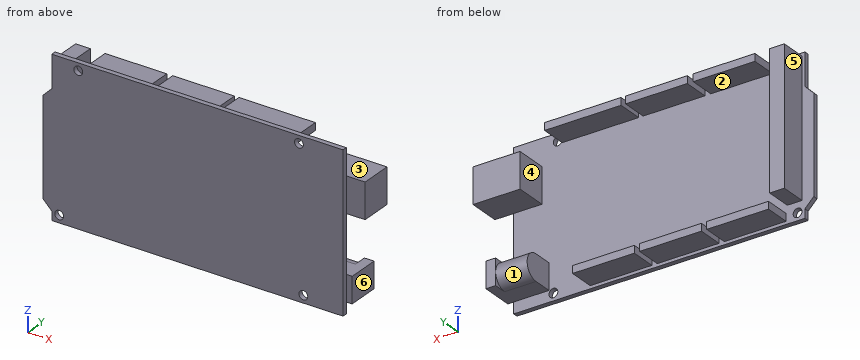
Autodesk Inventor part; units mm, degrees
ref_plane "YZ Plane" through (0, 0, 0) normal (1, 0, 0) x (0, 1, 0)
ref_plane "XZ Plane" through (0, 0, 0) normal (0, 1, 0) x (-1, 0, 0)
ref_plane "XY Plane" through (0, 0, 0) normal (0, 0, 1) x (1, 0, 0)
sketch "Sketch1" plane through (0, 0, 0) normal (0, 1, 0) x (-1, 0, 0)
  line L0 (0, 0) -> (99, 0)
  line L1 (99, 0) -> (99, 3)
  line L2 (99, 3) -> (102, 6)
  line L3 (102, 6) -> (102, 39)
  line L4 (102, 39) -> (99, 42)
  line L5 (99, 42) -> (99, 53)
  line L6 (99, 53) -> (0, 53)
  line L7 (0, 53) -> (0, 0)
  dimension "d0" = 99
  dimension "d1" = 3
  dimension "d2" = 135
  dimension "d3" = 33
  dimension "d4" = 3
  dimension "d5" = 3
  dimension "d6" = 53
extrude "Extrusion1" add sketch "Sketch1" along normal blind 1.6
sketch "Sketch2" plane through (0, 1.6, 0) normal (0, 1, 0) x (1, 0, 0)
  line L0 (0, 0) -> (-99, 0)
  line L1 (0, -53) -> (0, 0)
  line L2 (2, -3.8) -> (-12, -3.8)
  line L3 (-12, -3.8) -> (-12, -12.6)
  line L4 (-12, -12.6) -> (2, -12.6)
  line L5 (2, -12.6) -> (2, -3.8)
  dimension "d9" = 8.8
  dimension "d10" = 2
  dimension "d11" = 3.8
  dimension "d12" = 14
extrude "Extrusion2" add sketch "Sketch2" along normal blind 10.8
sketch "Sketch3" plane through (-12, 1.6, 3.8) normal (-1, 0, 0) x (0, 0, 1)
  line L0 (8.8, 0) -> (0, 0)
  line L1 (8.8, 0) -> (8.8, 10.8)
  line L2 (0, 10.8) -> (8.8, 10.8)
  line L3 (0, 0) -> (0, 10.8)
  arc A0 (8.8, 6.4) -> (0, 6.4) centre (4.4, 6.4) ccw
  point P0 (-3.8, -1.6)
extrude "Extrusion3" cut sketch "Sketch3" against normal blind 10.7 contours A0 L2 L1 | L3 L2 A0
sketch "Sketch4" plane through (0, 1.6, 0) normal (0, 1, 0) x (1, 0, 0)
  line L0 (-99, -53) -> (0, -53)
  line L1 (0, -53) -> (0, -12.6)
  line L2 (-9.6, -32) -> (6.4, -32)
  line L3 (6.4, -32) -> (6.4, -44)
  line L4 (6.4, -44) -> (-9.6, -44)
  line L5 (-9.6, -44) -> (-9.6, -32)
  dimension "d17" = 16
  dimension "d18" = 12
  dimension "d19" = 6.4
  dimension "d20" = 9
extrude "Extrusion4" add sketch "Sketch4" along normal blind 10.8
sketch "Sketch5" plane through (0, 1.6, 0) normal (0, 1, 0) x (1, 0, 0)
  line L0 (0, -3.8) -> (0, 0)
  line L1 (0, 0) -> (-99, 0)
  line L2 (-26, -3.5) -> (-47, -3.5)
  line L3 (-47, -3.5) -> (-47, -1)
  line L4 (-47, -1) -> (-26, -1)
  line L5 (-26, -1) -> (-26, -3.5)
  line L6 (-48.8, -3.5) -> (-69.8, -3.5)
  line L7 (-69.8, -3.5) -> (-69.8, -1)
  line L8 (-69.8, -1) -> (-48.8, -1)
  line L9 (-48.8, -1) -> (-48.8, -3.5)
  line L10 (-71.6, -3.5) -> (-92.6, -3.5)
  line L11 (-92.6, -3.5) -> (-92.6, -1)
  line L12 (-92.6, -1) -> (-71.6, -1)
  line L13 (-71.6, -1) -> (-71.6, -3.5)
  dimension "d23" = 21
  dimension "d24" = 2.5
  dimension "d25" = 26
  dimension "d26" = 1
  dimension "d29" = 22.8
extrude "Extrusion5" add sketch "Sketch5" along normal blind 8.7
sketch "Sketch6" plane through (0, 1.6, 0) normal (0, 1, 0) x (1, 0, 0)
  line L0 (0, 0) -> (-99, 0)
  line L1 (-102, -6) -> (-102, -39)
  line L2 (-98, -6) -> (-93, -6)
  line L3 (-93, -6) -> (-93, -52)
  line L4 (-93, -52) -> (-98, -52)
  line L5 (-98, -52) -> (-98, -6)
  dimension "d36" = 46
  dimension "d37" = 5
  dimension "d38" = 4
  dimension "d39" = 6
extrude "Extrusion6" add sketch "Sketch6" along normal blind 8.7
sketch "Sketch7" plane through (0, 1.6, 0) normal (0, 1, 0) x (1, 0, 0)
  line L0 (-99, -42) -> (-99, -53)
  line L1 (-99, -53) -> (0, -53)
  line L2 (-88, -49.5) -> (-67, -49.5)
  line L3 (-67, -49.5) -> (-67, -52)
  line L4 (-67, -52) -> (-88, -52)
  line L5 (-88, -52) -> (-88, -49.5)
  line L6 (-65, -49.5) -> (-44, -49.5)
  line L7 (-44, -49.5) -> (-44, -52)
  line L8 (-44, -52) -> (-65, -52)
  line L9 (-65, -52) -> (-65, -49.5)
  line L10 (-42.5, -49.5) -> (-16.5, -49.5)
  line L11 (-16.5, -49.5) -> (-16.5, -52)
  line L12 (-16.5, -52) -> (-42.5, -52)
  line L13 (-42.5, -52) -> (-42.5, -49.5)
  dimension "d42" = 21
  dimension "d43" = 2.5
  dimension "d44" = 1
  dimension "d45" = 11
  dimension "d48" = 23
  dimension "d54" = 26
  dimension "d55" = 1
  dimension "d56" = 1.5
extrude "Extrusion7" add sketch "Sketch7" along normal blind 8.7
hole "Hole1" at (-96.5, 1.6, 2.5) direction (0, -1, 0) diameter 3 end through all
hole "Hole2" at (-90, 1.6, 50.5) direction (0, -1, 0) diameter 3 end through all
hole "Hole3" at (-13.5, 1.6, 2.5) direction (0, -1, 0) diameter 3 end through all
hole "Hole4" at (-15, 1.6, 50.447) direction (0, -1, 0) diameter 3 end through all
properties part number "ArduinoMega"
The listing builds one solid part. Answer for the finished solid, in the listing's coordinates (mm). Face numbers are marked on the shaded views. A direction names the side the tool comes from. Coordinates: 2 decimals unless noted, no trailing zeros. Write each loop counter-clockwise with the first axis right and the second up, starting at its lowest first coordinate (ties: lowest second). Pieces come first, ordered by that corner, then holes. Notation, with made-up numbers: (-3, 22) -> (55, 22) arc R10 ccw to (55, 35) -> close; hole circle Ø11 at (59.5, 30.5). An arc over 180 degrees is marked (long way). One line per question, with ' | ' between items.
1. Which of the six approach directions +Z, -Z, +X, -X, +Y, -Y give full straight-line access (tool end or side, diameter ignored) to the marked faces 1, 2 and 3?
Verdict:
face 1: +Y | face 2: +X, +Y | face 3: +Z, +X, +Y
2. Section B-B (z = 24) is taken. Determine the outline of the cut face in (x, y).
Verdict:
outline: (-102, 0) -> (0, 0) -> (0, 1.6) -> (-93, 1.6) -> (-93, 10.3) -> (-98, 10.3) -> (-98, 1.6) -> (-102, 1.6) -> close
3. Straight lines are drawn through the part: line 1 (X direction, y = 0.6, z = 50.5); line 2 (Z direction, x = -90, y = 1); line 3 (X direction, y = 0.55, z = 2.5). For each, find the intervals that lie inside material, in ascending order.
Verdict:
line 1: x = -99 to -91.5, -88.5 to -16.5, -13.5 to 0 | line 2: z = 0 to 49, 52 to 53 | line 3: x = -99 to -98, -95 to -15, -12 to 0
4. Given pin 1 Ø0.8 at (y, z) = (5.5, 51) entering from +X; pin 2 Ø0.8 at (y, z) = (7.5, 2.5) entering from +X; pin 3 Ø5.5 at (y, z) = (9, 40) entering from -X, each flat-ended and moving along its own axis, determine where each tip first touches the part or whether it passes through.
Verdict:
pin 1: stops at x = -16.5 | pin 2: stops at x = -26 | pin 3: stops at x = -98
5. For a pull along X with two mould halves and no side action, classify the marked faces 4, 5 and 6 as released by +X, released by -X, zero draft, split by the parting line, or undercut.
Verdict:
face 4: undercut | face 5: released by -X | face 6: released by +X
6. Section C-C (x = -25) is taken. Determine the outline of the cut face in (y, z), and give its area (3 significant figures).
Verdict:
outline: (0, 0) -> (1.6, 0) -> (1.6, 49.5) -> (10.3, 49.5) -> (10.3, 52) -> (1.6, 52) -> (1.6, 53) -> (0, 53) -> close | area: 107 mm^2
7. Section D-D (y = 4.5) is taken. State how many separate pieces and enclosed holes the cut face has, and give its area (3 significant figures).
Verdict:
separate pieces: 9 | enclosed holes: 0 | area: 873 mm^2
8. Section A-A (x = -90) is taken. Determine the outline of the cut face in (y, z).
Verdict:
outline: (0, 0) -> (1.6, 0) -> (1.6, 1) -> (10.3, 1) -> (10.3, 3.5) -> (1.6, 3.5) -> (1.6, 49) -> (0, 49) -> close; (0, 52) -> (1.6, 52) -> (1.6, 53) -> (0, 53) -> close
